```python
from build123d import *

# Parameters (mm, degrees)
SKETCH1_W                      = 142.142719433
SKETCH1_H                      = 25.841975708
BOSS_EXTRUDE1_DEPTH            = 4
SKETCH2_W                      = 10
SKETCH2_H                      = 7
SKETCH3_W                      = 10
SKETCH3_H                      = 7
F_3_1_3_1_DIAMETER_HOLE1_D     = 3.1
F_3_1_3_1_DIAMETER_HOLE1_DEPTH = 11
F_6_0_6_DIAMETER_HOLE1_D       = 6
CHAMFER1_SIZE                  = 1
FILLET1_R                      = 6


with BuildPart() as part:
    # Sketch1 → Boss-Extrude1 (new body)
    with BuildSketch(Plane(origin=(0, 0, -8.279012494), x_dir=(-1, 0, 0), z_dir=(0, 0, -1))):
        with Locations((-40.928641953, 22.079012221)):
            Rectangle(SKETCH1_W, SKETCH1_H)
    extrude(amount=-BOSS_EXTRUDE1_DEPTH)

    # Sketch2 → Revolve1 (revolve)
    with BuildSketch(Plane(origin=(0, 22.079011948, 0), x_dir=(1, 0, 0), z_dir=(0, 1, 0))):
        with Locations((-5.54, 11.779012494)):
            Rectangle(SKETCH2_W, SKETCH2_H)
    revolve(axis=Axis((-10.54, 22.079011948, -15.279012494), (0, 0, 1)))

    # Sketch3 → Revolve2 (revolve)
    with BuildSketch(Plane(origin=(0, 22.079011948, 0), x_dir=(1, 0, 0), z_dir=(0, 1, 0))):
        with Locations((97.397001672, 11.779012494)):
            Rectangle(SKETCH3_W, SKETCH3_H)
    revolve(axis=Axis((92.397001672, 22.079011948, -15.279012494), (0, 0, 1)))

    # Ø3.1 (3.1) Diameter Hole1
    with Locations(Plane.XY.offset(-4.279012494)):
        with Locations((40.928641952, 28.039506364), (40.928641952, 15.618518294), (58.227283905, 27.164012494), (23.63, 27.164011948), (-23.63, 27.164011948), (-23.63, 16.994011948), (23.63, 16.994011948), (58.227283905, 16.994012494), (105.487283905, 27.164012494), (105.487283905, 16.994012494)):
            Hole(F_3_1_3_1_DIAMETER_HOLE1_D / 2, depth=F_3_1_3_1_DIAMETER_HOLE1_DEPTH)

    # Ø6.0 (6) Diameter Hole1 (through all)
    with Locations(Plane(origin=(0, 0, -15.279012494), x_dir=(-1, 0, 0), z_dir=(0, 0, -1))):
        with Locations((-92.397001672, 22.079344118), (10.54, 22.079011948)):
            Hole(F_6_0_6_DIAMETER_HOLE1_D / 2)

    # Chamfer1
    chamfer1_edges = [part.edges().sort_by_distance(p)[0] for p in [
        (-20.54, 22.079011948, -8.279012494),
        (-20.54, 22.079011948, -15.279012494),
        (82.397001672, 22.079011948, -8.279012494),
        (82.397001672, 22.079011948, -15.279012494),
    ]]
    chamfer(chamfer1_edges, length=CHAMFER1_SIZE)

    # Fillet1
    fillet1_edges = [part.edges().sort_by_distance(p)[0] for p in [
        (112.000001669, 35.000000075, -6.279012494),
        (-30.142717764, 35.000000075, -6.279012494),
        (-30.142717764, 9.158024367, -6.279012494),
        (112.000001669, 9.158024367, -6.279012494),
    ]]
    fillet(fillet1_edges, radius=FILLET1_R)


solid = part.part
```
Input: part model. Units: mm. Frame: model coordinates. A direction names the side the tool comes from. Coordinates: 2 decimals unless noted, no trailing zeros. Loops run counter-clockwise (first coordinate to the right, second up) from the corner with the lowest first, then second, coordinate; pieces in that order, holes last. Notation, with made-up numbers: M -19,-6 L 29,-6 A17 cw 29,16 Z; hole C 83.5,71.5 d1. An arc over 180 degrees is marked long. Answer in a Markdown table with one row per item.
1. Reachability of faces 1 (the cylindrical face through (106.717, 16.051, -6.307)), 2 (the cylindrical face through (101.935, 25.083, -11.814)) from +Z, -Z, +X, -X, +Y, -Y: full face, straight path, thin tool, end or side. Return the list, or none.
Response:
| item | result |
|---|---|
| face 1 | +Z, -Z |
| face 2 | -Z |
2. Section B-B, the plane x = -10.54. Output: boundary loops of the cut face in (y, z).
Response:
| item | result |
|---|---|
| outline | M 9.16,-8.28 L 11.08,-8.28 L 12.08,-9.28 L 12.08,-14.28 L 13.08,-15.28 L 19.08,-15.28 L 19.08,-4.28 L 9.16,-4.28 Z; M 25.08,-15.28 L 31.08,-15.28 L 32.08,-14.28 L 32.08,-9.28 L 33.08,-8.28 L 35,-8.28 L 35,-4.28 L 25.08,-4.28 Z |
3. Section A-A, the plane x = 23.63. Output: boundary loops of the cut face in (y, z).
Response:
| item | result |
|---|---|
| outline | M 9.16,-8.28 L 15.44,-8.28 L 15.44,-4.28 L 9.16,-4.28 Z; M 18.54,-8.28 L 25.61,-8.28 L 25.61,-4.28 L 18.54,-4.28 Z; M 28.71,-8.28 L 35,-8.28 L 35,-4.28 L 28.71,-4.28 Z |
4. Section C-C, the plane z = -12. Output: boundary loops of the cut face in (x, y), then the cut area to 3 significant figures.
Response:
| item | result |
|---|---|
| outline | C -10.54,22.08 d20; C 92.4,22.08 d20; hole C -10.54,22.08 d6; hole C 92.4,22.08 d6 |
| area | 572 mm2 |
5. First-contact query: pin 1 (1 mm diameter, centred on x = 82.5, y = 21, fed in from -Z); pin 2 (13 mm diameter, centred on x = 5.5, y = 23, fed in from -Z); pin 3 (3.5 mm diameter, centred on x = 23.63, y = 27.16, fed in from -Z). Flat tips, straight axial feed; report the tip coordinate or a pass-through.
Response:
| item | result |
|---|---|
| pin 1 | stops at z = -14.82 |
| pin 2 | stops at z = -14.71 |
| pin 3 | stops at z = -8.28 |
6. Material intervals for line 1 (Y direction, x = -23.63, z = -5.75); line 2 (X direction, y = 27, z = -7.25); line 3 (Y direction, x = 100, z = -9), sorted ascending.
Response:
| item | result |
|---|---|
| line 1 | y = 9.16 to 15.44, 18.54 to 25.61, 28.71 to 35 |
| line 2 | x = -30.14 to -25.17, -22.09 to 22.09, 25.17 to 39.78, 42.08 to 56.69, 59.77 to 103.95, 107.03 to 112 |
| line 3 | y = 15.16 to 29 |
7. Section D-D, the plane z = -6.25. Count the separate pieces of the cut face and the enclosed holes in it, then the cut area to 3 significant figures.
Response:
| item | result |
|---|---|
| separate pieces | 1 |
| enclosed holes | 12 |
| area | 3,510 mm2 |
8. Draft query along Y for faces 3 (the cylindrical face through (110.289, 10.962, -6.251)), 4 (the cylindrical face through (59.776, 27.232, -6.307)), 5 (the cylindrical face through (110.289, 33.196, -6.251)). Return one class per face: pulls with the +Y half, pulls with the -Y half, needs draft (parallel to the pull), parting line crosses it, or undercut.
Response:
| item | result |
|---|---|
| face 3 | pulls with the -Y half |
| face 4 | undercut |
| face 5 | pulls with the +Y half |
